Autodesk Fusion 360 part; units mm, degrees
sketch "Sketch1" plane through (0, 0, 0) normal (0, 1, 0) x (1, 0, 0)
  line L0 (0, 0) -> (89.803, 0)
  line L1 (89.803, 0) -> (89.803, 89.803)
  line L2 (89.803, 89.803) -> (0, 89.803)
  line L3 (0, 89.803) -> (0, 0)
  dimension "d1" = 89.803
  dimension "d2" = 89.803
extrude "Extrude1" add sketch "Sketch1" along normal blind 25 makes body 1
sketch "Sketch4" plane through (0, 25, 0) normal (0, 1, 0) x (-1, 0, 0)
  line L0 (0, -89.803) -> (0, 0)
  line L1 (0, 0) -> (-89.803, 0)
  line L2 (-89.803, 0) -> (-89.803, -89.803)
  line L3 (-89.803, -89.803) -> (0, -89.803)
  line L4 (-78.303, -78.303) -> (-11.5, -78.303)
  line L5 (-11.5, -78.303) -> (-11.5, -11.5)
  line L6 (-11.5, -11.5) -> (-78.303, -11.5)
  line L7 (-78.303, -11.5) -> (-78.303, -78.303)
  line L8 (-78.303, -78.303) -> (-11.5, -11.5) construction
  line L9 (-11.5, -78.303) -> (-78.303, -11.5) construction
  point P0 (-44.9015, -44.9015)
  dimension "d10" = 66.803
  dimension "d11" = 66.803
extrude "Extrude3" cut sketch "Sketch4" against normal blind 50 contours L4 L5 L6 L7 bodies 1
fillet "Fillet2" radius 3 4 edges at (0, 12.5, 0) (89.803, 12.5, 0) (89.803, 12.5, -89.803) (0, 12.5, -89.803) on bodies 1
sketch "Sketch5" plane through (0, 25, 0) normal (0, 1, 0) x (-1, 0, 0)
  arc A0 (-3, -89.803) -> (0, -86.803) centre (-3, -86.803) ccw
  line L0 (0, -86.803) -> (0, -3)
  arc A1 (0, -3) -> (-3, 0) centre (-3, -3) ccw
  line L1 (-3, 0) -> (-86.803, 0)
  arc A2 (-86.803, 0) -> (-89.803, -3) centre (-86.803, -3) ccw
  line L2 (-89.803, -3) -> (-89.803, -86.803)
  arc A3 (-89.803, -86.803) -> (-86.803, -89.803) centre (-86.803, -86.803) ccw
  line L3 (-86.803, -89.803) -> (-3, -89.803)
  line L4 (-11.5, -78.303) -> (-78.303, -78.303)
  line L5 (-78.303, -78.303) -> (-78.303, -11.5)
  line L6 (-78.303, -11.5) -> (-11.5, -11.5)
  line L7 (-11.5, -11.5) -> (-11.5, -78.303)
copy_body "Body->Comp2" bodies 1 removing the originals makes body 2 in component "midbody2"
sketch "Sketch6" plane through (44.9015, 25, -44.9015) normal (0, 1, 0) x (-1, 0, 0)
  circle A0 centre (-40, 40) radius 3
  circle A1 centre (40, 40) radius 3
  circle A2 centre (-40, -40) radius 3
  circle A3 centre (40, -40) radius 3
  dimension "d15" = 6
  dimension "d16" = 6
  dimension "d17" = 6
  dimension "d18" = 6
extrude "Extrude1'" cut sketch "Sketch6" against normal blind 3 bodies 2 in component "midbody2"
sketch "Sketch7" plane through (0, 0, 0) normal (0, -1, 0) x (1, 0, 0)
  line L0 (78.303, -78.303) -> (11.5, -78.303)
  line L1 (11.5, -78.303) -> (11.5, -11.5)
  line L2 (11.5, -11.5) -> (78.303, -11.5)
  line L3 (78.303, -11.5) -> (78.303, -78.303)
  arc A0 (0, -86.803) -> (3, -89.803) centre (3, -86.803) ccw
  line L4 (3, -89.803) -> (86.803, -89.803)
  arc A1 (86.803, -89.803) -> (89.803, -86.803) centre (86.803, -86.803) ccw
  line L5 (89.803, -86.803) -> (89.803, -3)
  arc A2 (89.803, -3) -> (86.803, 0) centre (86.803, -3) ccw
  line L6 (86.803, 0) -> (3, 0)
  arc A3 (3, 0) -> (0, -3) centre (3, -3) ccw
  line L7 (0, -3) -> (0, -86.803)
sketch "Sketch8" plane through (44.9015, 0, -44.9015) normal (0, -1, 0) x (1, 0, 0)
  circle A0 centre (40, 40) radius 3
  circle A1 centre (40, -40) radius 3
  circle A2 centre (40, -40) radius 3
  circle A3 centre (-40, -40) radius 3
  circle A4 centre (-40, 40) radius 3
  point P0 (-37, -40)
  point P1 (-37, 40)
  dimension "d21" = 6
  dimension "d22" = 6
  dimension "d24" = 6
  dimension "d25" = 6
extrude "Extrude2" cut sketch "Sketch8" against normal blind 3 bodies 2 in component "midbody2"
sketch "Sketch9" plane through (0, 25, 0) normal (0, 1, 0) x (-1, 0, 0)
  line L0 (-89.803, -3) -> (-89.803, -86.803)
  line L1 (-89.803, -86.803) -> (-89.803, -3)
  line L2 (-86.803, -89.803) -> (-3, -89.803)
  line L3 (0, -86.803) -> (0, -3)
  line L4 (0, -3) -> (0, -86.803)
  line L5 (-3, 0) -> (-86.803, 0)
  line L6 (-86.803, 0) -> (-3, 0)
  line L7 (-75, -7.5) -> (-15, -7.5)
  line L8 (-7.5, -15) -> (-7.5, -75)
  line L9 (-10.5518, -82.303) -> (-78.7446, -82.303)
  line L10 (-82.303, -79.8784) -> (-82.303, -9.9962)
  line L11 (-82.303, -9.9962) -> (-82.303, -7.5)
  line L12 (-82.303, -7.5) -> (-75, -7.5)
  line L13 (-7.5, -15) -> (-7.5, -7.5)
  line L14 (-15, -7.5) -> (-7.5, -7.5)
  line L15 (-7.5, -75) -> (-7.5, -82.303)
  line L16 (-10.5518, -82.303) -> (-7.5, -82.303)
  line L17 (-78.7446, -82.303) -> (-82.303, -82.303)
  line L18 (-82.303, -79.8784) -> (-82.303, -82.303)
extrude "Extrude3'" cut sketch "Sketch9" against normal blind 300 bodies 2 in component "midbody2"
component "midbody2" placed x (1, 0, 0) y (0, 1, 0) z (0, 0, 1) at (0, 0, 0)
For this review, take the finished solid that the model builds, in its own axes (mm). A direction names the side the tool comes from. Give positions to 0.01 mm unless a question says otherwise; leave off trailing zeros. Write each loop counter-clockwise with the first axis right and the second up, starting at its lowest first coordinate (ties: lowest second). Pieces come first, ordered by that corner, then holes. Notation, with made-up numbers: M 32.5,-30 L 64.5,-30 A25 ccw 64.5,-3 Z; hole C 17,15.25 d2. An arc over 180 degrees is marked long. Answer as CSV lines item,"result".
1. For pin 1 (3 mm diameter, centred on x = 5, z = -6, fed in from +Y); pin 2 (7.5 mm diameter, centred on y = 18, z = -33, fed in from -X); pin 3 (3.5 mm diameter, centred on x = 84.9, z = -84.9, fed in from -Y), all flat-tipped, find the tip position at first contact; note any pin that passes through.
Findings:
pin 1,"stops at y = 22"
pin 2,"stops at x = 0"
pin 3,"stops at y = 3"
2. For faces 1 (the flat face through (5, 22, -5)), 2 (the cylindrical face through (88.901, 12.675, -0.855)), 3 (the flat face through (45, 13, -7.5)), 4 (the cylindrical face through (81.904, 1.479, -4.77)), list the 3-axis set-ups (+Z, -Z, +X, -X, +Y, -Y) from which the entire face can be reached by the end or side of a thin tool; tool diameter is ignored.
Findings:
face 1,"+Y"
face 2,"+Z, +X, +Y, -Y"
face 3,"+Y, -Y"
face 4,"-Y"
3. Draft analysis for pull direction Z (two halves, no side actions). For faces 5 (the cylindrical face through (5.55, 23.52, -87.83)), 6 (the flat face through (0, 12, -45)), 7 (the cylindrical face through (88.95, 12.68, -88.9)), state which applies: +Z half, -Z half, draft (parallel to the pull), parting line (faces both ways), or undercut.
Findings:
face 5,"undercut"
face 6,"draft"
face 7,"-Z half"
4. Consider section B-B, the plane x = 60. Write out the cut boundary in (y, z), then the cut area to 3 significant figures.
Findings:
outline,"M 0,-89.8 L 25,-89.8 L 25,-82.3 L 0,-82.3 Z; M 0,-7.5 L 25,-7.5 L 25,0 L 0,0 Z"
area,"375 mm2"
5. Consider section C-C, the plane y = 6.75. Write out the cut boundary in (x, z), then the cut area to 3 significant figures.
Findings:
outline,"M 0,-86.8 A3 ccw 3,-89.8 L 86.8,-89.8 A3 ccw 89.8,-86.8 L 89.8,-3 A3 ccw 86.8,0 L 3,0 A3 ccw 0,-3 Z; hole M 7.5,-82.3 L 82.3,-82.3 L 82.3,-7.5 L 7.5,-7.5 Z"
area,"2,460 mm2"
6. Wall thickness on line 1 (X direction, y = 21.25, z = -78); line 2 (Z direction, x = 28.5, y = 23): over which ranges is each line inside the solid? List them lowest first.
Findings:
line 1,"x = 0 to 7.5, 82.3 to 89.8"
line 2,"z = -89.8 to -82.3, -7.5 to 0"
7. Consider section A-A, the plane z = -20. Write out the cut boundary in (x, y).
Findings:
outline,"M 0,0 L 7.5,0 L 7.5,25 L 0,25 Z; M 82.3,0 L 89.8,0 L 89.8,25 L 82.3,25 Z"
